Part model, mm, in its own coordinate system. Face numbers are marked on the shaded views. A direction names the side the tool comes from. Coordinates: 2 decimals unless noted, no trailing zeros. Loops run counter-clockwise (first coordinate to the right, second up) from the corner with the lowest first, then second, coordinate; pieces in that order, holes last. Notation, with made-up numbers: M 84.5,-25.75 L 109.5,-25.75 A15 cw 109.5,-21.75 Z; hole C 26,76 d11. An arc over 180 degrees is marked long. Use a Markdown table: item, result. Add a question column.
1) Band-saw the part on C-C (x = 0.3). List the corners of the cut face in (y, z).
2) Wall check: probe 1 along X at (y, z) = (0.5, 0); probe 2 along Y at (x, z) = (2.55, 1.5); probe 3 along Z at (x, y) = (-0.8, 1.5). Give the ranges that are in metal, low to high. Write a range as from..to.
3) Tool access for the marked faces 5 and 6: list every direction of +Z, -Z, +X, -X, +Y, -Y with a clear straight run to the whole face (end or side of a thin tool).
4) Pull direction X, two halves, no side cores. Call the marked faces 1, 2, 3 and 4: released by +X, released by -X, zero draft, split by the parting line, or undercut.
5) Band-saw the part on D-D (y = 4.75). List the corners of the cut face in (x, z), plus the area to 3 significant figures.
6) Band-saw the part on A-A (y = 1.5). List the corners of the cut face in (x, z).
7) Pin check, flat tips, straight feed: pin 1 Ø1.5 at (x, z) = (1, 2.5) entering from +Y; pin 2 Ø1.5 at (x, y) = (2, 4.5) entering from -Z; pin 3 Ø1.5 at (x, z) = (0, -0.5) entering from -Y. Stop position of each tip, or through.
from build123d import *

# Parameters (mm, degrees)
SZKIC1_R                    = 1.5
DODANIE_WYCI_GNI_CIE1_DEPTH = 2.4


with BuildPart() as part:
    # Szkic1 → Dodanie-wyciągnięcie1 (new body)
    with BuildSketch(Plane(origin=(0, 0, 0), x_dir=(1, 0, 0), z_dir=(0, 1, 0))):
        Polygon((0, 3.175426481), (-2.75, 1.58771324), (-2.75, -1.58771324), (0, -3.175426481), (2.75, -1.58771324), (2.75, 1.58771324), align=None)
        with Locations(Location((0, 0, 0), (0, 0, 270))):
            Circle(SZKIC1_R, mode=Mode.SUBTRACT)
    extrude(amount=DODANIE_WYCI_GNI_CIE1_DEPTH)

    # Szkic3 → Obrót2 (revolve)
    with BuildSketch(Plane.XY, mode=Mode.PRIVATE) as obr_t2_sk:
        with BuildLine():
            Line((0, 7), (0, 2.4))
            Line((0, 2.4), (2.75, 2.4))
            Line((2.75, 2.4), (2.75, 4.25))
            ThreePointArc((2.75, 4.25), (1.944543648, 6.194543648), (0, 7))
        make_face()
    revolve(obr_t2_sk.sketch.rotate(Axis((0, 7, 0), (0, -1, 0)), 180), axis=Axis((0, 7, 0), (0, -1, 0)))


solid = part.part
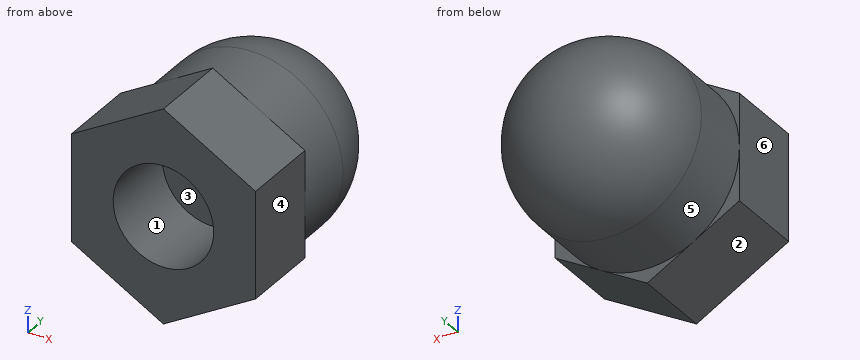
Entries:
| question | item | result |
|---|---|---|
| 1 | outline | M 0,-3 L 2.4,-3 L 2.4,-2.73 L 4.25,-2.73 A2.73 ccw 4.25,2.73 L 2.4,2.73 L 2.4,3 L 0,3 L 0,1.47 L 2.4,1.47 L 2.4,-1.47 L 0,-1.47 Z |
| 2 | probe 1 | -2.75..-1.5, 1.5..2.75 |
| 2 | probe 2 | 0..2.4 |
| 2 | probe 3 | -2.71..-1.27, 1.27..2.71 |
| 3 | face 5 | +Y |
| 3 | face 6 | +Z, -Z, -X, +Y, -Y |
| 4 | face 1 | undercut |
| 4 | face 2 | released by -X |
| 4 | face 3 | undercut |
| 4 | face 4 | released by +X |
| 5 | outline | C 0,0 d5.41 |
| 5 | area | 23.0 mm2 |
| 6 | outline | M -2.75,-1.59 L 0,-3.18 L 2.75,-1.59 L 2.75,1.59 L 0,3.18 L -2.75,1.59 Z; hole C 0,0 d3 |
| 7 | pin 1 | y = 6.2 |
| 7 | pin 2 | z = -2.44 |
| 7 | pin 3 | y = 2.4 |
